Read the model definition and answer for the solid it produces. Units are mm, in the model's axes. A direction names the side the tool comes from. Coordinates: 2 decimals unless noted, no trailing zeros. Loops run counter-clockwise (first coordinate to the right, second up) from the corner with the lowest first, then second, coordinate; pieces in that order, holes last. Notation, with made-up numbers: (-4, 55) - (8, 55) arc R20 cw to (8, 72) - close; hole circle Ø7 at (51, 37). An arc over 180 degrees is marked (long way). Use one line per item in the form item = value. Start each with the question number.
1) A cutting plane is placed at C-C (z = 1.15). Give the vertices of the cut face in (x, y), and give its area (3 significant figures).
2) A cutting plane is placed at D-D (x = 0). State how many separate pieces and enclosed holes the cut face has, and give its area (3 significant figures).
3) Which of the six approach directions +Z, -Z, +X, -X, +Y, -Y give full straight-line access (tool end or side, diameter ignored) to faces 5 (the face through (4, 0, 5)), 6 (the face through (5, 0, 1))?
4) The mould has two halves that part along Y. Classify faces 1 (the face through (-5, 0, 1)), 2 (the face through (0, 10, 3)), 3 (the face through (0, -10, 3)), 4 (the face through (3.233, -1.341, 3.231)): released by +Y, released by -Y, zero draft, split by the parting line, or undercut.
5) This flat-tipped pin is pushed along its axis until it touches: P1, Ø11, axis at x = -0.5, y = 1, coming from the -Z side. Where does it stop, or does it pass through?
6) Consider line 1 (Y direction, x = 0, z = 3.7); line 2 (X direction, y = 0.75, z = 1.1). Determine where each line is inside the solid, lowest interval first.
from build123d import *

# Parameters (mm, degrees)
F0_W     = 20
F0_H     = 20
F0_R     = 3.5
F1_DEPTH = 5
F2_W     = 10
F2_H     = 1.5
F3_DEPTH = 12.5


# Not quite as in the source:
# - a feature names something its author has since deleted; it is built from what else it names


with BuildPart() as f1:
    # F0 (on Top) → F1 (new body)
    with BuildSketch(Plane.XY):
        Rectangle(F0_W, F0_H)
        Circle(F0_R, mode=Mode.SUBTRACT)
    extrude(amount=F1_DEPTH)

    # F2 (on Front) → F3 (cut, symmetric)
    with BuildSketch(Plane.XZ):
        with Locations((0, 0.7610858302)):
            Rectangle(F2_W, F2_H)
    extrude(amount=F3_DEPTH, both=True, mode=Mode.SUBTRACT)


solid = f1.part
Found:
q1.outline = (-10, -10) - (-5, -10) - (-5, 10) - (-10, 10) - close; (5, -10) - (10, -10) - (10, 10) - (5, 10) - close
q1.area = 200 mm^2
q2.separate_pieces = 4
q2.enclosed_holes = 0
q2.area = 45.5 mm^2
q3.face_5 = +Z, +X, -X, +Y, -Y
q3.face_6 = +Y, -Y
q4.face_1 = zero draft
q4.face_2 = released by +Y
q4.face_3 = released by -Y
q4.face_4 = undercut
q5.P1 = 0
q6.line_1 = -10 to -3.5, 3.5 to 10
q6.line_2 = -10 to -5, 5 to 10
